from build123d import *

# Parameters (mm, degrees)
F0_W     = 20
F0_H     = 190
F0_R     = 2.5
F1_DEPTH = 10
F2_W     = 190
F2_H     = 5
F3_DEPTH = 15
F4_W     = 5
F4_H     = 190
F5_DEPTH = 30


with BuildPart() as f1:
    # F0 (on Top) → F1 (new body)
    with BuildSketch(Plane.XY):
        with Locations((0, 46.986108)):
            Rectangle(F0_W, F0_H)
        with Locations((0, -28.013892)):
            Circle(F0_R, mode=Mode.SUBTRACT)
        with Locations((0, 21.986108)):
            Circle(F0_R, mode=Mode.SUBTRACT)
        with Locations((0, 71.986108)):
            Circle(F0_R, mode=Mode.SUBTRACT)
        with Locations((0, 121.986108)):
            Circle(F0_R, mode=Mode.SUBTRACT)
    extrude(amount=F1_DEPTH)

    # F2 (on face) → F3 (join)
    with BuildSketch(Plane(origin=(-10, 0, 0), x_dir=(0, -1, 0), z_dir=(-1, 0, 0))):
        with Locations((-46.986108, 7.5)):
            Rectangle(F2_W, F2_H)
    extrude(amount=F3_DEPTH)

    # F4 (on face) → F5 (join)
    with BuildSketch(Plane.XY.offset(10)):
        with Locations((-17.5, 46.986108)):
            Rectangle(F4_W, F4_H)
    extrude(amount=F5_DEPTH)


solid = f1.part
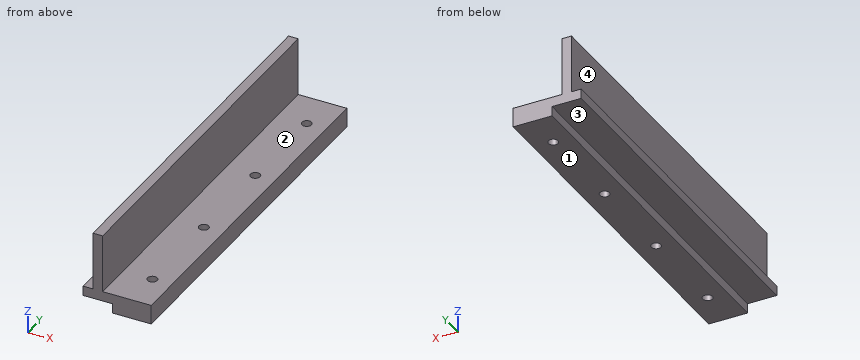
Part model, mm, in its own coordinate system. Face numbers are marked on the shaded views. A direction names the side the tool comes from. Round coordinates to 2 decimals unless told otherwise and drop trailing zeros. Write each loop counter-clockwise with the first axis right and the second up, starting at its lowest first coordinate (ties: lowest second). Pieces come first, ordered by that corner, then holes. Notation, with made-up numbers: (1.25, -20.75) - (57.25, -20.75) arc R15 cw to (57.25, 3.25) - close; hole circle Ø2 at (38.25, 9.5). An arc over 180 degrees is marked (long way). Use CSV: the item, a comma, the result in double quotes.
Item 1: Wall check: L1, parallel to Y at x = 0, z = 6; L2, parallel to Z at x = -4, y = 101; L3, parallel to X at y = 63, z = 29. Give the ranges that are in metal, low to high.
Results list:
L1,"y = -48.01 to -30.51, -25.51 to 19.49, 24.49 to 69.49, 74.49 to 119.49, 124.49 to 141.99"
L2,"z = 0 to 10"
L3,"x = -20 to -15"
Item 2: Flat gauge pins, fed straight in: P1, Ø8, axis at x = 0, y = 121.99, coming from the +Z side; P2, Ø1.5, axis at y = 86.5, z = 31, coming from the -X side; P3, Ø5.5, axis at y = 4.5, z = 1.5, coming from the -X side. Where does each tip first touch, or does it go through?
Results list:
P1,"stops at z = 10"
P2,"stops at x = -20"
P3,"stops at x = -10"
Item 3: Slice it at C-C, the plane z = 12.5. Write the cut outline in (x, y).
Results list:
outline,"(-20, -48.01) - (-15, -48.01) - (-15, 141.99) - (-20, 141.99) - close"
Item 4: Tool access for the marked faces 1, 2, 3 and 4: list every direction of +Z, -Z, +X, -X, +Y, -Y with a clear straight run to the whole face (end or side of a thin tool).
Results list:
face 1,"-Z, +X, -X, +Y, -Y"
face 2,"+Z, +X, +Y, -Y"
face 3,"-Z, -X, +Y, -Y"
face 4,"+Z, -X, +Y, -Y"
Item 5: Slice it at B-B, the plane y = 36. Write the cut outline in (x, z), then the cut area to 3 significant figures.
Results list:
outline,"(-25, 5) - (-10, 5) - (-10, 0) - (10, 0) - (10, 10) - (-15, 10) - (-15, 40) - (-20, 40) - (-20, 10) - (-25, 10) - close"
area,"425 mm²"
Item 6: Slice it at A-A, the plane x = 0. Write the cut outline in (y, z), then the cut area to 3 significant figures.
Results list:
outline,"(-48.01, 0) - (-30.51, 0) - (-30.51, 10) - (-48.01, 10) - close; (-25.51, 0) - (19.49, 0) - (19.49, 10) - (-25.51, 10) - close; (24.49, 0) - (69.49, 0) - (69.49, 10) - (24.49, 10) - close; (74.49, 0) - (119.49, 0) - (119.49, 10) - (74.49, 10) - close; (124.49, 0) - (141.99, 0) - (141.99, 10) - (124.49, 10) - close"
area,"1,700 mm²"
